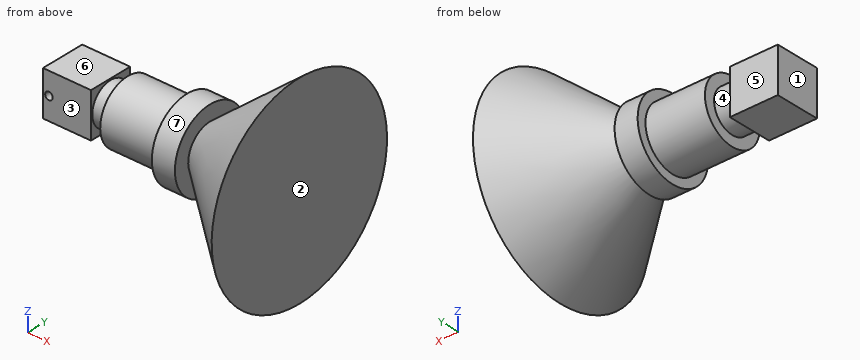
from build123d import *

# Parameters (mm, degrees)
SKETCH2_W                       = 32.25
SKETCH2_H                       = 30
BOSS_EXTRUDE1_DEPTH             = 15
SKETCH4_R                       = 14
BOSS_EXTRUDE2_DEPTH             = 11.5
SKETCH5_R                       = 21
BOSS_EXTRUDE3_DEPTH             = 40
SKETCH6_R                       = 27
BOSS_EXTRUDE4_DEPTH             = 15.5
TAP_DRILL_FOR_1_4_20_TAP1_D     = 5.1054
TAP_DRILL_FOR_1_4_20_TAP1_DEPTH = 4.76
TAP_DRILL_FOR_1_4_20_TAP1_TIP   = 1.533816902


with BuildPart() as part:
    # Sketch2 → Boss-Extrude1 (new, symmetric)
    with BuildSketch(Plane(origin=(0, 0, 0), x_dir=(1, 0, 0), z_dir=(0, 1, 0))):
        Rectangle(SKETCH2_W, SKETCH2_H)
    extrude(amount=BOSS_EXTRUDE1_DEPTH, both=True)

    # Sketch4 → Boss-Extrude2 (add)
    with BuildSketch(Plane(origin=(16.125, 0, 0), x_dir=(0, 0, -1), z_dir=(1, 0, 0))):
        Circle(SKETCH4_R)
    extrude(amount=BOSS_EXTRUDE2_DEPTH)

    # Sketch5 → Boss-Extrude3 (add)
    with BuildSketch(Plane(origin=(27.625, 0, 0), x_dir=(0, 0, -1), z_dir=(1, 0, 0))):
        Circle(SKETCH5_R)
    extrude(amount=BOSS_EXTRUDE3_DEPTH)

    # Sketch6 → Boss-Extrude4 (add)
    with BuildSketch(Plane(origin=(67.625, 0, 0), x_dir=(0, 0, -1), z_dir=(1, 0, 0))):
        Circle(SKETCH6_R)
    extrude(amount=BOSS_EXTRUDE4_DEPTH)

    # Sketch12 → Revolve1 (revolve)
    with BuildSketch(Plane.XY, mode=Mode.PRIVATE) as revolve1_sk:
        Polygon((63.125, 0), (143.125, 67.127970494), (143.125, 0), align=None)
    revolve(revolve1_sk.sketch.rotate(Axis((63.125, 0, 0), (1, 0, 0)), 270), axis=Axis((63.125, 0, 0), (1, 0, 0)))

    # Tap Drill for 1/4-20 Tap1
    with Locations(Plane(origin=(0, -15, 0), x_dir=(-1, 0, 0), z_dir=(0, -1, 0))):
        with Locations((12.125, 0)):
            Hole(TAP_DRILL_FOR_1_4_20_TAP1_D / 2, depth=TAP_DRILL_FOR_1_4_20_TAP1_DEPTH)
            with Locations((0, 0, -(TAP_DRILL_FOR_1_4_20_TAP1_DEPTH + TAP_DRILL_FOR_1_4_20_TAP1_TIP / 2))):  # 118° drill point
                Cone(0, TAP_DRILL_FOR_1_4_20_TAP1_D / 2, TAP_DRILL_FOR_1_4_20_TAP1_TIP, mode=Mode.SUBTRACT)


solid = part.part
Verification items for the finished model (mm, model axes). Face numbers are marked on the shaded views. A direction names the side the tool comes from. Coordinates: 2 decimals unless noted, no trailing zeros. Write each loop counter-clockwise with the first axis right and the second up, starting at its lowest first coordinate (ties: lowest second). Pieces come first, ordered by that corner, then holes. Notation, with made-up numbers: M 77,74.5 L 87,74.5 A14 ccw 87,99.5 Z; hole C 76,52.5 d7. An arc over 180 degrees is marked long. Use CSV: the item, a comma, the result in double quotes.
Q1. Section check A-A, the plane y = 0. Enter the section's corners in (x, z) (3 decimals), and give its area (3 significant figures).
Computed values:
outline,"M -16.125,-15 L 16.125,-15 L 16.125,-14 L 27.625,-14 L 27.625,-21 L 67.625,-21 L 67.625,-27 L 83.125,-27 L 83.125,-16.782 L 143.125,-67.128 L 143.125,67.128 L 83.125,16.782 L 83.125,27 L 67.625,27 L 67.625,21 L 27.625,21 L 27.625,14 L 16.125,14 L 16.125,15 L -16.125,15 Z"
area,"8,840 mm²"
Q2. Go/stop test with flat-tipped pins: P1, Ø12, axis at y = 46, z = 3, coming from the -X side; P2, Ø24, axis at x = 2.5, z = 6, coming from the -Y side; P3, Ø4, axis at x = -12.125, z = 0, coming from the -Y side. Record where each tip stops, or that it passes through.
Computed values:
P1,"x = 110.91"
P2,"y = -15"
P3,"y = -9.91"
Q3. Section check D-D, the plane x = 124. Enter the section's corners in (y, z).
Computed values:
outline,"C 0,0 d102.16"
Q4. Section check C-C, the plane x = 36.5. Enter the section's corners in (y, z), and give its area (3 significant figures).
Computed values:
outline,"C 0,0 d42"
area,"1,390 mm²"
Q5. Section check B-B, the plane x = 7. Enter the section's corners in (y, z).
Computed values:
outline,"M -15,-15 L 15,-15 L 15,15 L -15,15 Z"
Q6. Mould release check, pull along X, two halves, no side actions. Record for the marked faces 1, 2, 3 and 4: pulls with the +X half, pulls with the -X half, needs draft (parallel to the pull), parting line crosses it, or undercut.
Computed values:
face 1,"pulls with the -X half"
face 2,"pulls with the +X half"
face 3,"needs draft"
face 4,"undercut"
Q7. Thickness scan on line 1 along Y through (x, z) = (2, 10); line 2 along Z through (x, y) = (94, 21.5); line 3 along Z through (x, y) = (110, 4). Record the ranges inside material, lowest first. Write a range as [from, to].
Computed values:
line 1,"[-15, 15]"
line 2,"[-14.45, 14.45]"
line 3,"[-39.13, 39.13]"
Q8. Set-up check for the marked faces 5, 6 and 7: record each of +Z, -Z, +X, -X, +Y, -Y from which the full face is reachable in a straight line by a thin tool's end or side.
Computed values:
face 5,"+Z, -Z, -X, +Y"
face 6,"+Z, -X, +Y, -Y"
face 7,"-X"
